```python
from build123d import *

# Parameters (mm, degrees)
F1_DEPTH = 52
F2_R     = 11.0802059784
F2_R_2   = 11
F3_DEPTH = 51.6
F4_R     = 25.99999


# Not quite as in the source:
# - a fillet or chamfer is up to 0.001 mm smaller than in the source, because OpenCascade refuses the exact size


with BuildPart() as f1:
    # F0 (on Top) → F1 (new body)
    with BuildSketch(Plane.XY):
        with BuildLine():
            Line((109, 38), (-10.670231831, 38))
            ThreePointArc((-10.670231831, 38), (-92.7348286497, 70.2818364741), (-146, 0))
            Line((-146, 0), (-115, 0))
            ThreePointArc((-115, 0), (-73, 42), (-31, 0))
            Line((-31, 0), (109, 0))
            Line((109, 0), (109, 38))
        make_face()
    extrude(amount=F1_DEPTH)

    # F2 (on face) → F3 (cut)
    with BuildSketch(Plane.XZ):
        with Locations((35, 26)):
            Circle(F2_R)
        with Locations((83, 26)):
            Circle(F2_R_2)
    extrude(amount=-F3_DEPTH, mode=Mode.SUBTRACT)

    # F4 (radius 26 in the source; OpenCascade refuses exactly that, so slightly less here)
    f4_edges = [f1.edges().sort_by_distance(p)[0] for p in [
        (109, 19, 52),
        (109, 19, 0),
    ]]
    fillet(f4_edges, radius=F4_R)

    # F5 (on face) → F6 (revolve, cut)
    with BuildSketch(Plane.XZ):
        Polygon((-75.0884139538, 52), (-135.0884139538, 52), (-117.0884139538, 0), (-75.0884139538, 0), align=None)
    revolve(axis=Axis((-75.0884139538, 0, 26), (0, 0, 1)), mode=Mode.SUBTRACT)


solid = f1.part
```
Model file for the job. Use its own axes, mm. A direction names the side the tool comes from. Coordinates: 2 decimals unless noted, no trailing zeros. Order: outer loops, then holes, each group sorted by start corner. A loop starts at its lowest first (then second) coordinate and runs counter-clockwise, first axis right, second up. Notation, with made-up numbers: (59, 20) -> (108, 20) arc R24 cw to (108, 50) -> close; hole circle Ø2 at (85, -38). An arc over 180 degrees is marked (long way). Answer as a JSON object with one key per item and string values. Group by question number.
1) Cut at C-C, the plane y = 25.5. Count the separate pieces of the cut face and the enclosed holes in it, then the cut area to 3 significant figures.
2) Pull direction X, two halves, no side cores. Call faces 1 (the face through (101.59, 19.27, 7.82)), 2 (the face through (-91.455, 70.629, 25.636)), 3 (the face through (72, 19, 26)), 4 (the face through (-8, 29, 52)): +X half, -X half, draft (parallel to the pull), parting line (faces both ways), or undercut.
3) Which spindle directions (+Z, -Z, +X, -X, +Y, -Y) get a long thin tool onto all of the face, cutting with end or side? Do faces 5 (the face through (-39.105, 24.802, 2.304)), 6 (the face through (50, 38, 26)), 7 (the face through (38, 0, 14)). Say none if no direction does.
4) Drill centre lines: L1, parallel to X at y = 7.5, z = 35; L2, parallel to X at y = 10.5, z = 17.5; L3, parallel to Z at x = 35, y = 14.5. Where is each one in solid material? Low to high.
5) Flat gauge pins, fed straight in: pin 1 (12 mm diameter, centred on x = 82, z = 8, fed in from +Y); pin 2 (3 mm diameter, centred on y = 61.5, z = 45, fed in from -X); pin 3 (13.5 mm diameter, centred on x = 35, z = 26, fed in from +Y); pin 4 (1 mm diameter, centred on x = -68.5, z = 28.5, fed in from +Y). Where does each tip first touch, or does it go through?
6) Cut at B-B, the plane z = 30. Write the cut outline in (x, y).
7) Cut at A-A, the plane x = 35. Write the cut outline in (y, z), then the cut area to 3 significant figures.
8) Cut at D-D, the plane z = 45. Write the cut outline in (x, y).
Check values:
{
 "1": {"separate pieces": "2", "enclosed holes": "2", "area": "7,380 mm²"},
 "2": {"face 1": "+X half", "face 2": "parting line", "face 3": "undercut", "face 4": "draft"},
 "3": {"face 5": "+Z, -Z, -Y", "face 6": "+Z, -Z, +X, +Y", "face 7": "+Z, -Z, +X, -X, -Y"},
 "4": {"L1": "x = -145.61 to -128.68, -21.5 to 28.54, 41.46 to 76.68, 89.32 to 107.39", "L2": "x = -145.24 to -121.99, -28.19 to 27.89, 42.11 to 76.02, 89.98 to 107.57", "L3": "z = 0 to 14.92, 37.08 to 52"},
 "5": {"pin 1": "stops at y = 38", "pin 2": "stops at x = -114.58", "pin 3": "passes through", "pin 4": "stops at y = 72.89"},
 "6": {"outline": "(-146, 0) -> (-127.47, 0) arc R52.38 cw to (-22.7, 0) -> (24.67, 0) -> (24.67, 38) -> (-10.67, 38) arc R73 ccw to start; (45.33, 0) -> (72.75, 0) -> (72.75, 38) -> (45.33, 38) -> close; (93.25, 0) -> (108.69, 0) -> (108.69, 38) -> (93.25, 38) -> close"},
 "7": {"outline": "(0, 0) -> (38, 0) -> (38, 14.92) -> (0, 14.92) -> close; (0, 37.08) -> (38, 37.08) -> (38, 52) -> (0, 52) -> close", "area": "1,130 mm²"},
 "8": {"outline": "(-146, 0) -> (-132.67, 0) arc R57.58 cw to (-17.51, 0) -> (100.75, 0) -> (100.75, 38) -> (-10.67, 38) arc R73 ccw to start"}
}
